CAD build for the part. Positions are in the model's coordinates, mm. A direction names the side the tool comes from. Round coordinates to 2 decimals unless told otherwise and drop trailing zeros. Write each loop counter-clockwise with the first axis right and the second up, starting at its lowest first coordinate (ties: lowest second). Pieces come first, ordered by that corner, then holes. Notation, with made-up numbers: (-29.5, -1.75) -> (-9.5, -1.75) arc R18 ccw to (-9.5, 23.25) -> close; hole circle Ø1 at (38, 67). An arc over 180 degrees is marked (long way). Put each result on its own line as item: value. Start each with the question number.
1. 3-axis set-ups, long thin cutter, end or side, ignore diameter. For faces 1 (the flat face through (1786, -508, 690.005)), 2 (the flat face through (1761.3, -568, 562)): which of +Z, -Z, +X, -X, +Y, -Y reach the whole face in a straight line?
2. Saw through at C-C on y = -499.5. List the corners of the cut face in (x, z) (3 decimals).
3. Saw through at B-B on z = 583. List the corners of the cut face in (x, y) (3 decimals), and give its area (3 significant figures).
4. Drill centre lines: line 1 (Y direction, x = 1786.7, z = 693.25) (3 decimals); line 2 (Z direction, x = 1799.4, y = -566) (3 decimals); line 3 (Y direction, x = 1786, z = 691) (3 decimals). Where is each one in solid material? Low to high. Write a range as from..to.
5. Flat gauge pins, fed straight in: P1, Ø8.5, axis at x = 1786.7, z = 551.855, coming from the -Y side; P2, Ø3, axis at x = 1774, y = -500.5, coming from the -Z side (3 decimals). Where does each tip first touch, or does it go through?
6. Pull direction X, two halves, no side cores. Call faces 3 (the cylindrical face through (1803.416, -567.284, 346.302)), 4 (the flat face through (1786, -452.495, 693)), 5 (the flat face through (1812.1, -568, 562)): pulls with the +X half, pulls with the -X half, needs draft (parallel to the pull), parting line crosses it, or undercut.
7. Saw through at A-A on x = 1799.4. List the corners of the cut face in (y, z) (3 decimals).
from build123d import *

# Parameters (mm, degrees)
CROQUIS2_W              = 50.8
CROQUIS2_H              = 6.31
CROQUIS3_W              = 50.8
CROQUIS3_H              = 6.31
CROQUIS4_W              = 60
CROQUIS4_H              = 53.155
SALIENTE_EXTRUIR1_DEPTH = 6.31
CROQUIS5_W              = 60
CROQUIS5_H              = 6.31
CORTAR_EXTRUIR1_DEPTH   = 6.31
CORTAR_EXTRUIR2_DEPTH   = 634
CROQUIS8_W              = 50.8
CROQUIS8_H              = 6.31
SALIENTE_EXTRUIR2_DEPTH = 63.5
CROQUIS9_R              = 5
CORTAR_EXTRUIR3_DEPTH   = 10
CROQUIS10_W             = 790.847933
CROQUIS10_H             = 6.31
CORTAR_EXTRUIR4_DEPTH   = 286
CROQUIS11_W             = 50.8
CROQUIS11_H             = 6.31
CROQUIS11_W_2           = 210
CORTAR_EXTRUIR5_DEPTH   = 13.11
CROQUIS12_W             = 50.8
CROQUIS12_H             = 6.31
SALIENTE_EXTRUIR3_DEPTH = 6.35
CROQUIS13_W             = 50.8
CROQUIS13_H             = 6.35
CORTAR_EXTRUIR6_DEPTH   = 6.35
CROQUIS14_W             = 260.8
CROQUIS14_H             = 6.31
CORTAR_EXTRUIR7_DEPTH   = 6.31
CROQUIS15_W             = 50.8
CROQUIS15_H             = 6.31
CORTAR_EXTRUIR8_DEPTH   = 6.31
CROQUIS16_W             = 78.776397836
CROQUIS16_H             = 454.479218284
CORTAR_EXTRUIR9_DEPTH   = 128
CROQUIS22_R             = 4.7625
CORTAR_EXTRUIR15_DEPTH  = 33
CROQUIS24_R             = 5.000000022
CORTAR_EXTRUIR18_DEPTH  = 33
CROQUIS25_R             = 4.7625
CORTAR_EXTRUIR19_DEPTH  = 50


with BuildPart() as part:
    # Barrer1: sweep along a curve in space
    with BuildLine() as barrer1_path:
        Line((0, 0, 0), (0, -567.24, 0))
        Line((0, -567.24, 0), (0, -567.24, 336.2))
        Line((0, -567.24, 336.2), (1786.7, -567.24, 336.2))
        Line((1786.7, -567.24, 336.2), (1786.7, -567.24, 693.16))
        Line((1786.7, -567.24, 693.16), (1786.7, -436.23, 693.16))
        Line((1786.7, -436.23, 693.16), (1786.7, -436.23, 1487.162933))
    # Croquis2 → Barrer1 (sweep)
    with BuildSketch(Plane(origin=(0, 0, 0), x_dir=(1, 0, 0), z_dir=(0, 1, 0))):
        Rectangle(CROQUIS2_W, CROQUIS2_H)
        with Locations((210, 0)):
            Rectangle(CROQUIS2_W, CROQUIS2_H)
    sweep(path=barrer1_path.line, transition=Transition.RIGHT)

    # Barrer4: sweep along a curve in space
    with BuildLine() as barrer4_path:
        Line((-0.201028049, -3.155, -3.155), (-0.201028049, -3.155, -207.155))
        Line((-0.201028049, -3.155, -207.155), (-0.201028049, -53.155, -207.155))
    # Croquis3 → Barrer4 (sweep)
    with BuildSketch(Plane(origin=(0, 0, -3.155), x_dir=(-1, 0, 0), z_dir=(0, 0, -1))):
        with Locations((-210, -3.155)):
            Rectangle(CROQUIS3_W, CROQUIS3_H)
        with Locations((0, -3.155)):
            Rectangle(CROQUIS3_W, CROQUIS3_H)
    sweep(path=barrer4_path.line, transition=Transition.RIGHT)

    # Croquis4 → Saliente-Extruir1 (add)
    with BuildSketch(Plane(origin=(0, 0, -210.31), x_dir=(-1, 0, 0), z_dir=(0, 0, -1))):
        with Locations((-154.6, -26.5775)):
            Rectangle(CROQUIS4_W, CROQUIS4_H)
    extrude(amount=-SALIENTE_EXTRUIR1_DEPTH)

    # Croquis5 → Cortar-Extruir1 (cut)
    with BuildSketch(Plane.XY.offset(-204)):
        with Locations((154.6, -3.155)):
            Rectangle(CROQUIS5_W, CROQUIS5_H)
    extrude(amount=-CORTAR_EXTRUIR1_DEPTH, mode=Mode.SUBTRACT)

    # Croquis7 → Cortar-Extruir2 (cut)
    with BuildSketch(Plane(origin=(0, 0, 0), x_dir=(1, 0, 0), z_dir=(0, 1, 0))):
        Polygon((1761.3, -361.6), (2022.1, -361.6), (2022.1, 278.600557529), (-188.115947115, 278.600557529), (-188.115947115, -361.6), align=None)
    extrude(amount=-CORTAR_EXTRUIR2_DEPTH, mode=Mode.SUBTRACT)

    # Croquis8 → Saliente-Extruir2 (add)
    with BuildSketch(Plane(origin=(0, 0, 361.6), x_dir=(-1, 0, 0), z_dir=(0, 0, -1))):
        with Locations((-1786.7, -567.24)):
            Rectangle(CROQUIS8_W, CROQUIS8_H)
    extrude(amount=SALIENTE_EXTRUIR2_DEPTH)

    # Croquis9 → Cortar-Extruir3 (cut)
    with BuildSketch(Plane(origin=(0, -433.075, 0), x_dir=(1, 0, 0), z_dir=(0, 1, 0))):
        with Locations(Location((1786.7, -1454.162933, 0), (0, 0, 270))):
            Circle(CROQUIS9_R)
        with Locations(Location((1786.7, -1234.162933, 0), (0, 0, 270))):
            Circle(CROQUIS9_R)
        with Locations(Location((1996.7, -1234.162933, 0), (0, 0, 270))):
            Circle(CROQUIS9_R)
        with Locations(Location((1996.7, -1454.162933, 0), (0, 0, 270))):
            Circle(CROQUIS9_R)
    extrude(amount=-CORTAR_EXTRUIR3_DEPTH, mode=Mode.SUBTRACT)

    # Croquis10 → Cortar-Extruir4 (cut)
    with BuildSketch(Plane(origin=(2022.1, 0, 0), x_dir=(0, 0, -1), z_dir=(1, 0, 0))):
        with Locations((-1091.7389665, -436.23)):
            Rectangle(CROQUIS10_W, CROQUIS10_H)
    extrude(amount=-CORTAR_EXTRUIR4_DEPTH, mode=Mode.SUBTRACT)

    # Croquis11 → Cortar-Extruir5 (cut)
    with BuildSketch(Plane(origin=(0, -433.075, 0), x_dir=(1, 0, 0), z_dir=(0, 1, 0))):
        with Locations((1996.7, -693.16)):
            Rectangle(CROQUIS11_W, CROQUIS11_H)
        with Locations((1866.3, -693.16)):
            Rectangle(CROQUIS11_W_2, CROQUIS11_H)
    extrude(amount=-CORTAR_EXTRUIR5_DEPTH, mode=Mode.SUBTRACT)

    # Croquis12 → Saliente-Extruir3 (add)
    with BuildSketch(Plane(origin=(0, 0, 361.6), x_dir=(-1, 0, 0), z_dir=(0, 0, -1))):
        with Locations((-1996.7, -567.24)):
            Rectangle(CROQUIS12_W, CROQUIS12_H)
    extrude(amount=SALIENTE_EXTRUIR3_DEPTH)

    # Croquis13 → Cortar-Extruir6 (cut)
    with BuildSketch(Plane(origin=(0, -564.085, 0), x_dir=(1, 0, 0), z_dir=(0, 1, 0))):
        with Locations((1786.7, -301.275)):
            Rectangle(CROQUIS13_W, CROQUIS13_H)
    extrude(amount=-CORTAR_EXTRUIR6_DEPTH, mode=Mode.SUBTRACT)

    # Croquis14 → Cortar-Extruir7 (cut)
    with BuildSketch(Plane(origin=(0, -446.185, 0), x_dir=(1, 0, 0), z_dir=(0, 1, 0))):
        with Locations((1891.7, -693.16)):
            Rectangle(CROQUIS14_W, CROQUIS14_H)
    extrude(amount=-CORTAR_EXTRUIR7_DEPTH, mode=Mode.SUBTRACT)

    # Croquis15 → Cortar-Extruir8 (cut)
    with BuildSketch(Plane(origin=(0, 0, 304.45), x_dir=(-1, 0, 0), z_dir=(0, 0, -1))):
        with Locations((-1786.7, -567.24)):
            Rectangle(CROQUIS15_W, CROQUIS15_H)
    extrude(amount=-CORTAR_EXTRUIR8_DEPTH, mode=Mode.SUBTRACT)

    # Croquis16 → Cortar-Extruir9 (cut)
    with BuildSketch(Plane(origin=(0, -452.495, 0), x_dir=(1, 0, 0), z_dir=(0, 1, 0))):
        with Locations((1993.809618139, -557.908989907)):
            Rectangle(CROQUIS16_W, CROQUIS16_H)
    extrude(amount=-CORTAR_EXTRUIR9_DEPTH, mode=Mode.SUBTRACT)

    # Croquis22 → Cortar-Extruir15 (cut)
    with BuildSketch(Plane(origin=(0, -564.085, 0), x_dir=(1, 0, 0), z_dir=(0, 1, 0))):
        with Locations(Location((1786.7, -551.855, 0), (0, 0, 270))):
            Circle(CROQUIS22_R)
    extrude(amount=-CORTAR_EXTRUIR15_DEPTH, mode=Mode.SUBTRACT)

    # Croquis24 → Cortar-Extruir18 (cut)
    with BuildSketch(Plane(origin=(0, 0, 690.005), x_dir=(-1, 0, 0), z_dir=(0, 0, -1))):
        with Locations((-1786.700000078, -486.49871274)):
            Circle(CROQUIS24_R)
    extrude(amount=-CORTAR_EXTRUIR18_DEPTH, mode=Mode.SUBTRACT)

    # Croquis25 → Cortar-Extruir19 (cut)
    with BuildSketch(Plane(origin=(0, -570.395, 0), x_dir=(-1, 0, 0), z_dir=(0, -1, 0))):
        with Locations(Location((-1799.399999999, -348.862204666, 0), (0, 0, 90))):
            Circle(CROQUIS25_R)
        with Locations(Location((-1773.999999999, -323.462204666, 0), (0, 0, 90))):
            Circle(CROQUIS25_R)
    extrude(amount=-CORTAR_EXTRUIR19_DEPTH, mode=Mode.SUBTRACT)


solid = part.part
Return value:
1. face 1: -Z, +X, -X, +Y
1. face 2: +Z, -Z, -X, +Y, -Y
2. outline: (1761.3, 690.005) -> (1812.1, 690.005) -> (1812.1, 696.315) -> (1761.3, 696.315) -> close
3. outline: (1761.3, -570.395) -> (1812.1, -570.395) -> (1812.1, -564.085) -> (1761.3, -564.085) -> close
3. area: 321 mm^2
4. line 1: y = -570.395..-491.499, -481.499..-452.495
4. line 2: z = 310.76..344.1, 353.625..696.315
4. line 3: y = -570.395..-491.449, -481.548..-452.495
5. P1: passes through
5. P2: stops at z = 690.005
6. face 3: undercut
6. face 4: needs draft
6. face 5: pulls with the +X half
7. outline: (-570.395, 310.76) -> (-564.085, 310.76) -> (-564.085, 344.1) -> (-570.395, 344.1) -> close; (-570.395, 353.625) -> (-564.085, 353.625) -> (-564.085, 690.005) -> (-452.495, 690.005) -> (-452.495, 696.315) -> (-570.395, 696.315) -> close
